Geometry check sheet. Reference: drawing and pictorial views, mm from the part's lowest x, y, z. Round coordinates to 2 decimals unless told otherwise and drop trailing zeros. Order: outer loops, then holes, each group sorted by start corner. A loop starts at its lowest first (then second) coordinate and runs counter-clockwise, first axis right, second up.
Q1. Mould release check, pull along X, two halves, no side actions. Record for the marked faces 1, 2 and 3: +X half, -X half, draft (parallel to the pull), parting line (faces both ways), or undercut.
Q2. Cross-section at B-B on x = 25. Record the cut outline in (y, z) (1 decimal).
Q3. Depth check by flat-ended pin: P1, Ø4, axis at y = 27.5, z = 33, coming from the -X side; P2, Ø1.5, axis at x = 32, y = 18, coming from the -Z side; P3, Ø4, axis at x = 28.5, z = 80, coming from the -Y side; P4, Ø12, axis at y = 27.5, z = 55, coming from the +X side. Enter the tip coordinate at first touch or a pass-through.
Q4. Cross-section at D-D on x = 39. Record the cut outline in (y, z).
Q5. Scan lines: probe 1 along Y at (x, z) = (21, 96); probe 2 along Y at (x, z) = (9.5, 91.5) (1 decimal); probe 3 along Z at (x, y) = (30, 2.5). Record each from-to range of solid material in increasing order.
Q6. Cross-section at A-A on y = 19. Record the cut outline in (x, z).
Q7. Cross-section at C-C on z = 15. Record the cut outline in (x, y).
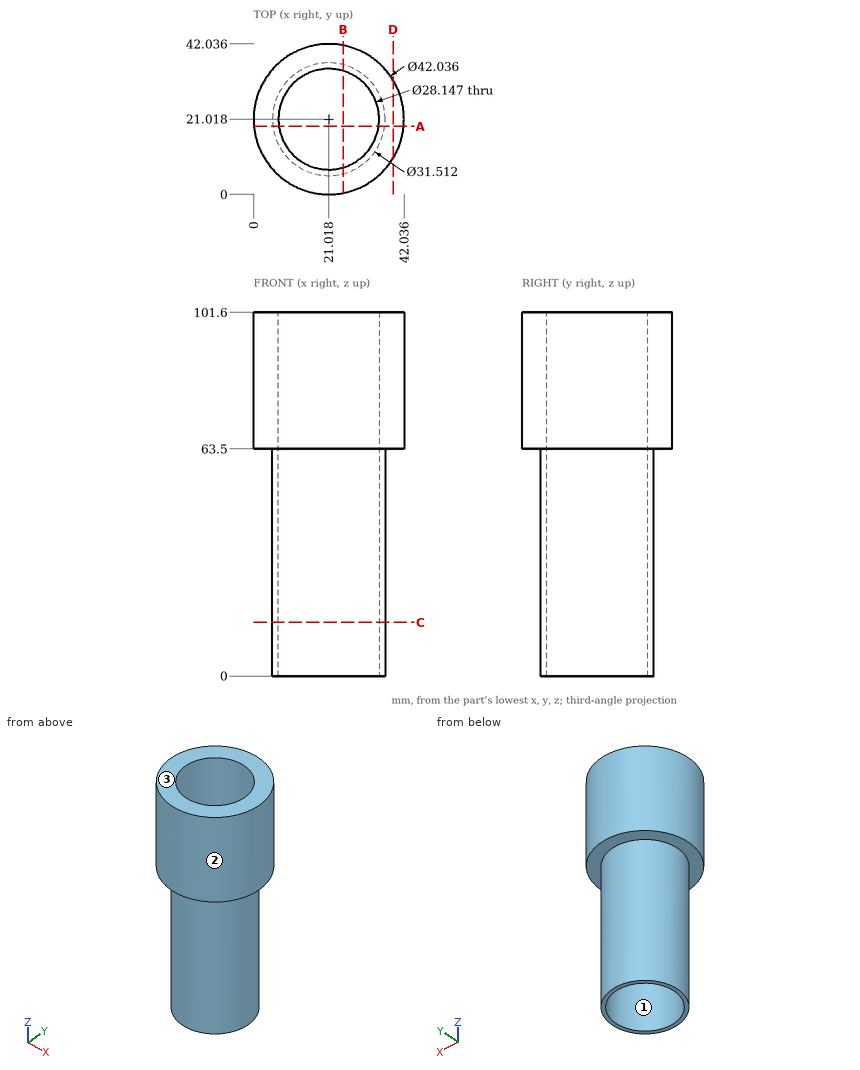
Results found:
1. face 1: undercut
1. face 2: parting line
1. face 3: draft
2. outline: (0.4, 63.5) - (5.8, 63.5) - (5.8, 0) - (7.5, 0) - (7.5, 101.6) - (0.4, 101.6) - close; (34.5, 0) - (36.3, 0) - (36.3, 63.5) - (41.7, 63.5) - (41.7, 101.6) - (34.5, 101.6) - close
3. P1: stops at x = 5.91
3. P2: passes through
3. P3: stops at y = 0.73
3. P4: stops at x = 36.77
4. outline: (10.14, 63.5) - (31.9, 63.5) - (31.9, 101.6) - (10.14, 101.6) - close
5. probe 1: y = 0 to 6.94, 35.09 to 42.04
5. probe 2: y = 3.4 to 12.9, 29.1 to 38.6
5. probe 3: z = 63.5 to 101.6
6. outline: (0.1, 63.5) - (5.39, 63.5) - (5.39, 0) - (7.09, 0) - (7.09, 101.6) - (0.1, 101.6) - close; (34.95, 0) - (36.64, 0) - (36.64, 63.5) - (41.94, 63.5) - (41.94, 101.6) - (34.95, 101.6) - close
7. outline: circle Ø31.51 at (21.02, 21.02); hole circle Ø28.15 at (21.02, 21.02)
